from build123d import *

# Parameters (mm, degrees)
F4_W        = 53
F4_H        = 35.5
F5_DEPTH    = 60
F6_T1_DEPTH = 60
F7_R        = 5.04
F9_T1_DEPTH = 74.3591672048
F10_T       = -2
F12_R       = 53
F13_R       = 2
F11_W       = 35
F11_H       = 21
F14_DEPTH   = 2
F15_R       = 3


# Not quite as in the source:
# - a fillet or chamfer that OpenCascade refuses, or shapes differently, is made with other operations: its cross-section is extruded or revolved along the edge and cut away or added
# - two fillets or chamfers of one size are made in one step


with BuildPart() as f5:
    # F4 (on Top) → F5 (new body)
    with BuildSketch(Plane.XY):
        with BuildLine():
            Line((-26.5, 0), (-26.5, -2))
            Line((-26.5, -2), (26.5, -2))
            Line((26.5, -2), (26.5, 0))
            Line((26.5, 0), (5.0951280026, 0))
            ThreePointArc((5.0951280026, 0), (0, -1), (-5.0951280026, 0))
            Line((-5.0951280026, 0), (-26.5, 0))
        make_face()
        with Locations((0, -19.75)):
            Rectangle(F4_W, F4_H)
        with BuildLine():
            ThreePointArc((-9.414110408, 22.1284476932), (-13.2305158305, 9.8978613101), (-5.0951280026, 0))
            Line((-5.0951280026, 0), (5.0951280026, 0))
            ThreePointArc((5.0951280026, 0), (13.2305158305, 9.8978613101), (9.414110408, 22.1284476932))
            ThreePointArc((9.414110408, 22.1284476932), (8.753655045, 22.7314262234), (8.0546720819, 23.2892857143))
            ThreePointArc((8.0546720819, 23.2892857143), (0, 1), (-8.0546720819, 23.2892857143))
            ThreePointArc((-8.0546720819, 23.2892857143), (-8.753655045, 22.7314262234), (-9.414110408, 22.1284476932))
        make_face()
        with BuildLine():
            Line((5.0951280026, 0), (-5.0951280026, 0))
            ThreePointArc((-5.0951280026, 0), (0, -1), (5.0951280026, 0))
        make_face()
        with BuildLine():
            Line((-9.414110408, 27.0511904762), (-9.414110408, 22.1284476932))
            ThreePointArc((-9.414110408, 22.1284476932), (-8.753655045, 22.7314262234), (-8.0546720819, 23.2892857143))
            Line((-8.0546720819, 23.2892857143), (-9.414110408, 27.0511904762))
        make_face()
        with BuildLine():
            ThreePointArc((8.0546720819, 23.2892857143), (8.753655045, 22.7314262234), (9.414110408, 22.1284476932))
            Line((9.414110408, 22.1284476932), (9.414110408, 27.0511904762))
            Line((9.414110408, 27.0511904762), (8.0546720819, 23.2892857143))
        make_face()
    extrude(amount=F5_DEPTH)

    # F6: fillet of radius 126 on 2 edges, made by hand

    # F6_s2 → F6_t1 (join)
    with BuildSketch(Plane.XY):
        with BuildLine():
            ThreePointArc((-9.414110408, 27.0511904762), (-10.9216954082, 22.0848726308), (-12.632526933, 17.1848541647))
            ThreePointArc((-12.632526933, 17.1848541647), (-11.297049781, 19.8348574754), (-9.414110408, 22.1284476932))
            Line((-9.414110408, 22.1284476932), (-9.414110408, 27.0511904762))
        make_face()
        with BuildLine():
            ThreePointArc((12.632526933, 17.1848541647), (10.9216954082, 22.0848726308), (9.414110408, 27.0511904762))
            Line((9.414110408, 27.0511904762), (9.414110408, 22.1284476932))
            ThreePointArc((9.414110408, 22.1284476932), (11.297049781, 19.8348574754), (12.632526933, 17.1848541647))
        make_face()
    extrude(amount=F6_T1_DEPTH)

    # F7
    f7_edges = [f5.edges().sort_by_distance(p)[0] for p in [
        (-5.095128, 0, 30),
        (5.095128, 0, 30),
        (8.054672, 23.289286, 30),
        (-8.054672, 23.289286, 30),
    ]]
    fillet(f7_edges, radius=F7_R)

    # F9: fillet of radius 5.04 on 2 edges, made by hand

    # F9_s2 → F9_t1 (cut)
    with BuildSketch(Plane.XY.offset(-7.1795836024)):
        with BuildLine():
            ThreePointArc((10.2229827876, 24.2956228784), (9.778060574, 25.324045565), (9.116903363, 26.2287444879))
            Line((9.116903363, 26.2287444879), (9.414110408, 27.0511904762))
            ThreePointArc((9.414110408, 27.0511904762), (9.8106956175, 25.6711020918), (10.2229827876, 24.2956228784))
        make_face()
        with BuildLine():
            ThreePointArc((-10.2229827876, 24.2956228784), (-9.778060574, 25.324045565), (-9.116903363, 26.2287444879))
            Line((-9.116903363, 26.2287444879), (-9.414110408, 27.0511904762))
            ThreePointArc((-9.414110408, 27.0511904762), (-9.8106956175, 25.6711020918), (-10.2229827876, 24.2956228784))
        make_face()
    extrude(amount=F9_T1_DEPTH, mode=Mode.SUBTRACT)

    # F10
    f10_openings = [f5.faces().sort_by_distance(p)[0] for p in [
        (0, -17.249718, 60),
    ]]
    offset(amount=F10_T, openings=f10_openings)

    # F12
    f12_edges = [f5.edges().sort_by_distance(p)[0] for p in [
        (-10.182168, 3.136566, 31),
        (10.182168, 3.136566, 31),
    ]]
    fillet(f12_edges, radius=F12_R)

    # F13
    f13_edges = [f5.edges().sort_by_distance(p)[0] for p in [
        (-26.5, 0, 30),
        (26.5, 0, 30),
        (24.5, -35.5, 31),
        (-24.5, -35.5, 31),
        (26.5, -37.5, 30),
        (-26.5, -37.5, 30),
        (24.5, -2, 31),
        (-24.5, -2, 31),
    ]]
    fillet(f13_edges, radius=F13_R)

    # F11 (on face) → F14 (cut)
    with BuildSketch(Plane(origin=(0, 0, 0), x_dir=(1, 0, 0), z_dir=(0, 0, -1))):
        with Locations((0, 18.75)):
            Rectangle(F11_W, F11_H)
    extrude(amount=-F14_DEPTH, mode=Mode.SUBTRACT)

    # F15
    f15_edges = [f5.edges().sort_by_distance(p)[0] for p in [
        (17.5, -8.25, 1),
        (-17.5, -8.25, 1),
        (-17.5, -29.25, 1),
        (17.5, -29.25, 1),
    ]]
    fillet(f15_edges, radius=F15_R)


solid = f5.part
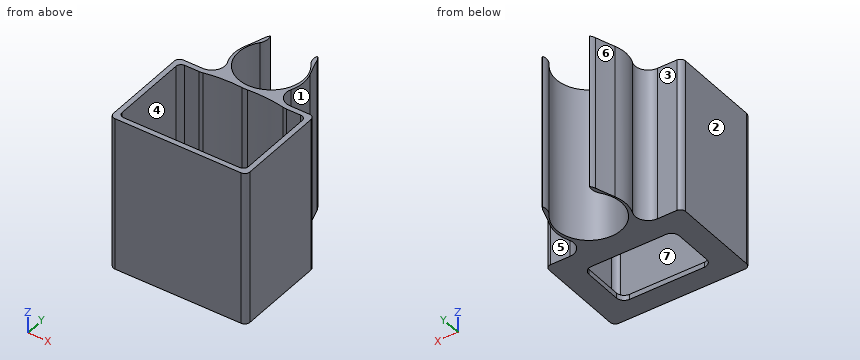
Model file for the job. Use its own axes, mm. Face numbers are marked on the shaded views. A direction names the side the tool comes from. Give positions to 0.01 mm unless a question says otherwise; leave off trailing zeros. Loops run counter-clockwise (first coordinate to the right, second up) from the corner with the lowest first, then second, coordinate; pieces in that order, holes last. Notation, with made-up numbers: (-8, -24) -> (46, -24) arc R15 cw to (46, -7) -> close; hole circle Ø1 at (42.25, 37). An arc over 180 degrees is marked (long way). Use a Markdown table: item, result. Add a question column.
(1) Slice it at C-C on y = 13.6. List the corners of the cut face in (x, z).
(2) Slice it at B-B on x = 19.5. List the corners of the cut face in (y, z).
(3) Wall check: line 1 along Y through (x, z) = (18.5, 42.5); line 2 along X through (y, z) = (-30.5, 48.5); line 3 along Y through (x, z) = (-0.5, 42). Give the ranges that are in metal, low to high.
(4) Slice it at A-A on x = 0. List the corners of the cut face in (y, z), and give its area (3 significant figures).
(5) Tool access for the marked faces 5, 6 and 7: list every direction of +Z, -Z, +X, -X, +Y, -Y with a clear straight run to the whole face (end or side of a thin tool).
(6) Mould opens along X. For the marked faces 1, 2, 3 and 4 say: +X half, -X half, draft (parallel to the pull), parting line (faces both ways), or undercut.
(7) Drop flat-ended pins along their axis: pin 1 Ø12 at (y, z) = (11.5, 18.5) entering from -X; pin 2 Ø4 at (x, y) = (-15, -30) entering from +Z; pin 3 Ø1.6 at (x, z) = (-5, 1) entering from +Y. Give the stop position or say it passes through.
Filled sheet:
| question | item | result |
|---|---|---|
| 1 | outline | (-13.43, 0) -> (-12.6, 0) -> (-12.6, 60) -> (-13.43, 60) -> close; (12.6, 0) -> (13.43, 0) -> (13.43, 60) -> (12.6, 60) -> close |
| 2 | outline | (-37.5, 0) -> (0, 0) -> (0, 60) -> (-2, 60) -> (-2, 2) -> (-35.5, 2) -> (-35.5, 60) -> (-37.5, 60) -> close |
| 3 | line 1 | -37.5 to -35.5, -2 to 0 |
| 3 | line 2 | -26.5 to -24.5, 24.5 to 26.5 |
| 3 | line 3 | -37.5 to -35.5, -0.99 to 1.01 |
| 4 | outline | (-37.5, 0) -> (-29.25, 0) -> (-29.25, 2) -> (-35.5, 2) -> (-35.5, 60) -> (-37.5, 60) -> close; (-8.25, 0) -> (1, 0) -> (1, 60) -> (-1, 60) -> (-1, 2) -> (-8.25, 2) -> close |
| 4 | area | 267 mm2 |
| 5 | face 5 | +Z, -Z, +X, +Y |
| 5 | face 6 | +Z, -Z, -X, +Y |
| 5 | face 7 | +Z |
| 6 | face 1 | +X half |
| 6 | face 2 | -X half |
| 6 | face 3 | draft |
| 6 | face 4 | undercut |
| 7 | pin 1 | x = -13.48 |
| 7 | pin 2 | z = 2 |
| 7 | pin 3 | y = 2.41 |
